Geometry: final body of the model. Coordinates: model frame, mm. Face numbers are marked on the shaded views. A direction names the side the tool comes from. Give positions to 0.01 mm unless a question says otherwise; leave off trailing zeros. Loops run counter-clockwise (first coordinate to the right, second up) from the corner with the lowest first, then second, coordinate; pieces in that order, holes last.
from build123d import *

# Parameters (mm, degrees)
F3_R = 6
F4_R = 9.5


# Not quite as in the source:
# - a fillet or chamfer that OpenCascade refuses, or shapes differently, is made with other operations: its cross-section is extruded or revolved along the edge and cut away or added


with BuildPart() as f1:
    # F0 (on Front) → F1 (revolve)
    with BuildSketch(Plane.XZ):
        Polygon((0, 4.5), (0, 0), (64, 0), (64, 9.5), (9, 9.5), (9, 4.5), align=None)
    revolve(axis=Axis((32, 0, 0), (1, 0, 0)))

    # F2: fillet of radius 8 on 1 edges, made by hand

    # F2_s1 → F2_t2 (revolve, cut)
    with BuildSketch(Plane.XZ):
        with BuildLine():
            ThreePointArc((16.4161984871, 9.5), (11.9440625321, 8.1332495807), (9, 4.5))
            Line((9, 4.5), (9, 9.5))
            Line((9, 9.5), (16.4161984871, 9.5))
        make_face()
    revolve(axis=Axis((9, 0, 0), (1, 0, 0)), mode=Mode.SUBTRACT)

    # F3
    f3_edges = [f1.edges().sort_by_distance(p)[0] for p in [
        (9, 0, -4.5),
    ]]
    fillet(f3_edges, radius=F3_R)

    # F4
    f4_edges = [f1.edges().sort_by_distance(p)[0] for p in [
        (64, 0, -9.5),
    ]]
    fillet(f4_edges, radius=F4_R)


solid = f1.part
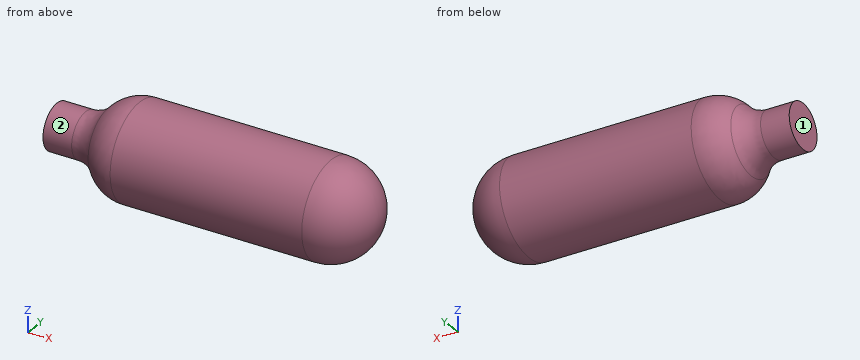
Item 1: Set-up query: the marked faces 1 and 2. Return all of +Z, -Z, +X, -X, +Y, -Y with unobstructed straight access to the full face (end or side cutting, diameter ignored); none if empty.
Values follow:
face 1: +Z, -Z, -X, +Y, -Y
face 2: -X
Item 2: Section query A-A on x = 27.5. Return loops of the section in (y, z).
Values follow:
outline: circle Ø19 at (0, 0)
Item 3: Pin query (flat end, axial travel): pin 1 (3 mm diameter, centred on y = -5, z = 1.5, fed in from +X); pin 2 (10 mm diameter, centred on x = 8.5, y = 4, fed in from +Z); pin 3 (6 mm diameter, centred on x = 56, z = 7.5, fed in from -Y) (3 decimals). Return the tip coordinate at first contact, or that it passes through.
Values follow:
pin 1: stops at x = 63.24
pin 2: stops at z = 8.54
pin 3: stops at y = -8.285
Item 4: Ray query, probe 1 along Z at (x, y) = (54, -0.5); probe 2 along Z at (x, y) = (24, 7); probe 3 along X at (y, z) = (-5.75, -3.25). Return the intervals inside material, ascending.
Values follow:
probe 1: z = -9.49 to 9.49
probe 2: z = -6.42 to 6.42
probe 3: x = 10.26 to 61.33
